Autodesk Inventor part; units mm, degrees
ref_plane "YZ Plane" through (0, 0, 0) normal (1, 0, 0) x (0, 1, 0)
ref_plane "XZ Plane" through (0, 0, 0) normal (0, 1, 0) x (-1, 0, 0)
ref_plane "XY Plane" through (0, 0, 0) normal (0, 0, 1) x (1, 0, 0)
sketch "Náčrt1" plane through (0, 0, 0) normal (0, 0, 1) x (1, 0, 0)
  line L0 (0, 0) -> (600, 0)
  line L1 (600, 0) -> (600, -180)
  line L2 (600, -180) -> (0, -180)
  line L3 (0, -180) -> (0, 0)
  line L4 (0, -80) -> (220, 0)
  dimension "d43" = 600
  dimension "d44" = 180
  dimension "d45" = 100
  dimension "d46" = 220
extrude "Vysunutí1" add sketch "Náčrt1" against normal blind 180 contours L0 L1 L2 L3 L4
sketch "Náčrt6" plane through (600, -180, 0) normal (1, 0, 0) x (0, 0, -1)
  line L0 (180, 180) -> (180, 0)
  line L1 (0, 0) -> (0, 180)
  line L2 (180, 180) -> (0, 0) construction
  circle A0 centre (90, 90) radius 65
  dimension "d47" = 130
extrude "Vysunutí6" add sketch "Náčrt6" along normal blind 30
sketch "Náčrt7" plane through (0, -180, 0) normal (0, -1, 0) x (1, 0, 0)
  circle A0 centre (100, -90) radius 50
  line L0 (0, 0) -> (0, -180)
  line L1 (0, -90) -> (285.9708, -90) construction
  dimension "d50" = 100
  dimension "d51" = 100
extrude "Vysunutí7" cut sketch "Náčrt7" against normal blind 10
sketch "Náčrt8" plane through (100, -170, -90) normal (0, -1, 0) x (1, 0, 0)
  circle A0 centre (0, 0) radius 20
  point P0 (-100, 90)
  dimension "d54" = 40
extrude "Vysunutí8" add sketch "Náčrt8" along normal blind 70
sketch "Náčrt5" plane through (0, 0, 0) normal (0, 0, 1) x (-1, 0, 0)
  circle A0 centre (0, 0) radius 65
  dimension "d40" = 130
properties part number "B7-A3"
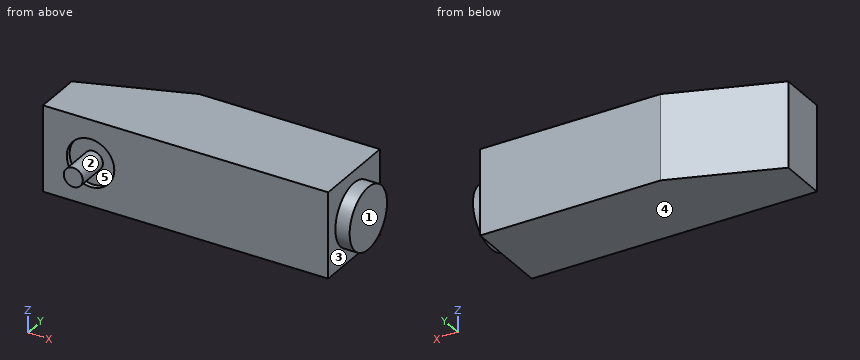
Could you check a few things on this model? Use its own coordinates, in mm. Face numbers are marked on the shaded views. A direction names the side the tool comes from. Give positions to 0.01 mm unless a question says otherwise; leave off trailing zeros. Order: outer loops, then holes, each group sorted by start corner. A loop starts at its lowest first (then second) coordinate and runs counter-clockwise, first axis right, second up.
Item 1: For the marked faces 1 and 2, which set-ups out of +Z, -Z, +X, -X, +Y, -Y let a thin tool reach every point of the face, with its end or its side?
Item 2: If we section it at B-B, the plane z = -90: Write out the boundary of the cut face in (x, y), plus the area to 3 significant figures.
Item 3: I'm going to push flat-ended pins straight in: pin 1 (2 mm diameter, centred on x = 301, y = -120.5, fed in from +Z); pin 2 (2 mm diameter, centred on x = 117, y = -190, fed in from -Z). Where does each tip first touch, or does it pass through?
Item 4: If we section it at D-D, the plane z = -15: Write out the boundary of the cut face in (x, y).
Item 5: If we section it at C-C, the plane x = 144: Write out the boundary of the cut face in (y, z), plus the area to 3 significant figures.
Item 6: If we section it at A-A, the plane y = -51: Write out the boundary of the cut face in (x, z).
Item 7: I need wall thicknesses on line 1 (Z direction, x = 100, y = -173); line 2 (Y direction, x = 512.5, z = -117); line 3 (X direction, y = -139, z = -22). Which ranges of each line are inside material? Lowest first, please.
Item 8: If we mould it in two halves opening along X, with no side actions, what happens to the marked faces 3, 4 and 5? For each: pulls with the +X half, pulls with the -X half, needs draft (parallel to the pull), parting line crosses it, or undercut.
Values:
1. face 1: +Z, -Z, +X, +Y, -Y
1. face 2: -Y
2. outline: (0, -180) - (50, -180) - (50, -170) - (80, -170) - (80, -240) - (120, -240) - (120, -170) - (150, -170) - (150, -180) - (600, -180) - (600, -155) - (630, -155) - (630, -25) - (600, -25) - (600, 0) - (220, 0) - (0, -80) - close
2. area: 105,000 mm2
3. pin 1: stops at z = 0
3. pin 2: stops at z = -102
4. outline: (0, -180) - (600, -180) - (600, 0) - (220, 0) - (0, -80) - close
5. outline: (-180, -180) - (-27.64, -180) - (-27.64, 0) - (-180, 0) - (-180, -66.25) - (-170, -66.25) - (-170, -113.75) - (-180, -113.75) - close
5. area: 27,000 mm2
6. outline: (79.75, -180) - (600, -180) - (600, -142) - (630, -142) - (630, -38) - (600, -38) - (600, 0) - (79.75, 0) - close
7. line 1: z = -180 to -140, -110 to -70, -40 to 0
7. line 2: y = -180 to 0
7. line 3: x = 0 to 600
8. face 3: pulls with the +X half
8. face 4: needs draft
8. face 5: undercut
